```python
from build123d import *

# Parameters (mm, degrees)
F0_R     = 17.5
F1_DEPTH = 80
F3_DEPTH = 63.5


with BuildPart() as f1:
    # F0 (on Top) → F1 (new body)
    with BuildSketch(Plane.XY):
        Circle(F0_R)
    extrude(amount=F1_DEPTH)

    # F2 (on face) → F3 (cut)
    with BuildSketch(Plane.XY.offset(80)):
        with BuildLine():
            Line((4.25, -14.4989), (4.25, -9.3273790531))
            ThreePointArc((4.25, -9.3273790531), (0, -10.25), (-4.25, -9.3273790531))
            Line((-4.25, -9.3273790531), (-4.25, -14.4989))
            Line((-4.25, -14.4989), (4.25, -14.4989))
        make_face()
        with BuildLine():
            ThreePointArc((4.25, -9.3273790531), (8.6204698248, -5.5452682532), (10.25, 0))
            ThreePointArc((10.25, 0), (8.6204698248, 5.5452682532), (4.25, 9.3273790531))
            Line((4.25, 9.3273790531), (4.25, -9.3273790531))
        make_face()
        with BuildLine():
            Line((4.25, -9.3273790531), (4.25, 9.3273790531))
            ThreePointArc((4.25, 9.3273790531), (0, 10.25), (-4.25, 9.3273790531))
            Line((-4.25, 9.3273790531), (-4.25, -9.3273790531))
            ThreePointArc((-4.25, -9.3273790531), (0, -10.25), (4.25, -9.3273790531))
        make_face()
        with BuildLine():
            Line((-4.25, -9.3273790531), (-4.25, 9.3273790531))
            ThreePointArc((-4.25, 9.3273790531), (-10.25, 0), (-4.25, -9.3273790531))
        make_face()
    extrude(amount=-F3_DEPTH, mode=Mode.SUBTRACT)


solid = f1.part
```
Design review of the part built by this model. Coordinates are the model's own, in mm. A direction names the side the tool comes from. Coordinates: 2 decimals unless noted, no trailing zeros. Loops run counter-clockwise (first coordinate to the right, second up) from the corner with the lowest first, then second, coordinate; pieces in that order, holes last.
Q1. We need section B-B on x = 0. State the section outline as (y, z) points, and give its area (3 significant figures).
Reported:
outline: (-17.5, 0) - (17.5, 0) - (17.5, 80) - (10.25, 80) - (10.25, 16.5) - (-14.5, 16.5) - (-14.5, 80) - (-17.5, 80) - close
area: 1,230 mm2
Q2. For pin 1 (6 mm diameter, centred on x = 0, y = -7, fed in from +Z); pin 2 (3 mm diameter, centred on y = -2, z = 71.5, fed in from -X); pin 3 (1.5 mm diameter, centred on x = -8.5, z = 28, fed in from +Y), all flat-tipped, find the tip position at first contact; note any pin that passes through.
Reported:
pin 1: stops at z = 16.5
pin 2: stops at x = -17.49
pin 3: stops at y = 15.69
Q3. We need section A-A on z = 65. State the section outline as (x, y) points, and give its area (3 significant figures).
Reported:
outline: circle Ø35 at (0, 0); hole (-4.25, -14.5) - (4.25, -14.5) - (4.25, -9.33) arc R10.25 ccw (long way) to (-4.25, -9.33) - close
area: 593 mm2
Q4. To check wall thickness, follow line 1 (Y direction, x = 2, z = 48); line 2 (Y direction, x = -5.5, z = 75.5); line 3 (X direction, y = -8.5, z = 30.5). State the ranges of each line that lie inside material, in increasing order.
Reported:
line 1: y = -17.39 to -14.5, 10.05 to 17.39
line 2: y = -16.61 to -8.65, 8.65 to 16.61
line 3: x = -15.3 to -5.73, 5.73 to 15.3
Q5. We need section D-D on z = 12. State the section outline as (x, y) points, and give its area (3 significant figures).
Reported:
outline: circle Ø35 at (0, 0)
area: 962 mm2
Q6. We need section C-C on y = -1. State the section outline as (x, z) points.
Reported:
outline: (-17.47, 0) - (17.47, 0) - (17.47, 80) - (10.2, 80) - (10.2, 16.5) - (-10.2, 16.5) - (-10.2, 80) - (-17.47, 80) - close
Q7. Tool access review of faces 4 (the face through (0, 0, 0)), 5 (the face through (4.25, -12, 49)): name each direction out of +Z, -Z, +X, -X, +Y, -Y from which nothing blocks a thin tool from reaching the whole face with its end or side.
Reported:
face 4: -Z, +X, -X, +Y, -Y
face 5: +Z
Q8. The part is to be moulded in two halves that separate along Y. For faces 1 (the face through (8, 8, 80)), 2 (the face through (-13.887, -10.648, 39.44)), 3 (the face through (0, -14.499, 49)), say which applies: +Y half, -Y half, draft (parallel to the pull), parting line (faces both ways), or undercut.
Reported:
face 1: draft
face 2: parting line
face 3: undercut
